```python
from build123d import *

# Parameters (mm, degrees)
SKETCH_1_W      = 50
SKETCH_1_H      = 50
SKETCH_1_R      = 3.5
SKETCH_1_R_2    = 6
EXTRUDE_1_DEPTH = 4
FILLET_1_R      = 5


with BuildPart() as part:
    # 草图1 → 凸台-拉伸1 (new body)
    with BuildSketch(Plane.XY):
        Rectangle(SKETCH_1_W, SKETCH_1_H)
        with Locations((0, 14)):
            Circle(SKETCH_1_R, mode=Mode.SUBTRACT)
        with Locations((12.124355653, 7)):
            Circle(SKETCH_1_R, mode=Mode.SUBTRACT)
        with Locations((12.124355653, -7)):
            Circle(SKETCH_1_R, mode=Mode.SUBTRACT)
        with Locations((0, -14)):
            Circle(SKETCH_1_R, mode=Mode.SUBTRACT)
        with Locations((-12.124355653, -7)):
            Circle(SKETCH_1_R, mode=Mode.SUBTRACT)
        with Locations((-12.124355653, 7)):
            Circle(SKETCH_1_R, mode=Mode.SUBTRACT)
        Circle(SKETCH_1_R_2, mode=Mode.SUBTRACT)
    extrude(amount=EXTRUDE_1_DEPTH)

    # 圆角1
    fillet_1_edges = [part.edges().sort_by_distance(p)[0] for p in [
        (-25, 25, 2),
        (25, 25, 2),
        (25, -25, 2),
        (-25, -25, 2),
    ]]
    fillet(fillet_1_edges, radius=FILLET_1_R)


solid = part.part
```
Can you work these out from the model? Positions are in its coordinate system, mm. Coordinates: 2 decimals unless noted, no trailing zeros. Loops run counter-clockwise (first coordinate to the right, second up) from the corner with the lowest first, then second, coordinate; pieces in that order, holes last. Notation, with made-up numbers: M 62.25,66 L 118.25,66 A18 ccw 118.25,79 Z; hole C -8,79.25 d9. An arc over 180 degrees is marked long. Put each result on its own line as item: value. Start each with the question number.
(1) Imagine slicing it at A-A on y = -14. List the corners of the cut face in (x, z) for me, and give its area (3 significant figures).
(2) We'd pull the mould along X, two halves only. Please class faces 1 (the face through (23, 24, 2)), 2 (the face through (-0.759, 10.583, 1.972)), 3 (the face through (11.366, -10.417, 1.972)), 4 (the face through (0, -25, 2)): +X half, -X half, draft (parallel to the pull), parting line (faces both ways), or undercut.
(3) Imagine slicing it at C-C on z = 1.1. List the corners of the cut face in (x, y) for me, and give its area (3 significant figures).
(4) Imagine slicing it at D-D on y = 7. List the corners of the cut face in (x, z) for me.
(5) Will these pins go through, and if not, where does the flat tip stop? pin 1 Ø11 at (x, y) = (12.12, 7) entering from -Z; pin 2 Ø6.5 at (x, y) = (-12.12, 7) entering from -Z.
(6) Imagine slicing it at B-B on x = 0. List the corners of the cut face in (y, z) for me.
(7) I need wall thicknesses on probe 1 along Y at (x, z) = (0, 1.65); probe 2 along Y at (x, z) = (13.5, 2.65); probe 3 along Y at (x, z) = (1, 0.7). Which ranges of each line are inside material? Lowest first, please.
Worked answers:
1. outline: M -25,0 L -3.5,0 L -3.5,4 L -25,4 Z; M 3.5,0 L 25,0 L 25,4 L 3.5,4 Z
1. area: 172 mm2
2. face 1: +X half
2. face 2: undercut
2. face 3: undercut
2. face 4: draft
3. outline: M -25,-20 A5 ccw -20,-25 L 20,-25 A5 ccw 25,-20 L 25,20 A5 ccw 20,25 L -20,25 A5 ccw -25,20 Z; hole C -12.12,-7 d7; hole C -12.12,7 d7; hole C 0,0 d12; hole C 0,-14 d7; hole C 0,14 d7; hole C 12.12,-7 d7; hole C 12.12,7 d7
3. area: 2,130 mm2
4. outline: M -25,0 L -15.62,0 L -15.62,4 L -25,4 Z; M -8.62,0 L 8.62,0 L 8.62,4 L -8.62,4 Z; M 15.62,0 L 25,0 L 25,4 L 15.62,4 Z
5. pin 1: stops at z = 0
5. pin 2: passes through
6. outline: M -25,0 L -17.5,0 L -17.5,4 L -25,4 Z; M -10.5,0 L -6,0 L -6,4 L -10.5,4 Z; M 6,0 L 10.5,0 L 10.5,4 L 6,4 Z; M 17.5,0 L 25,0 L 25,4 L 17.5,4 Z
7. probe 1: y = -25 to -17.5, -10.5 to -6, 6 to 10.5, 17.5 to 25
7. probe 2: y = -25 to -10.22, -3.78 to 3.78, 10.22 to 25
7. probe 3: y = -25 to -17.35, -10.65 to -5.92, 5.92 to 10.65, 17.35 to 25
